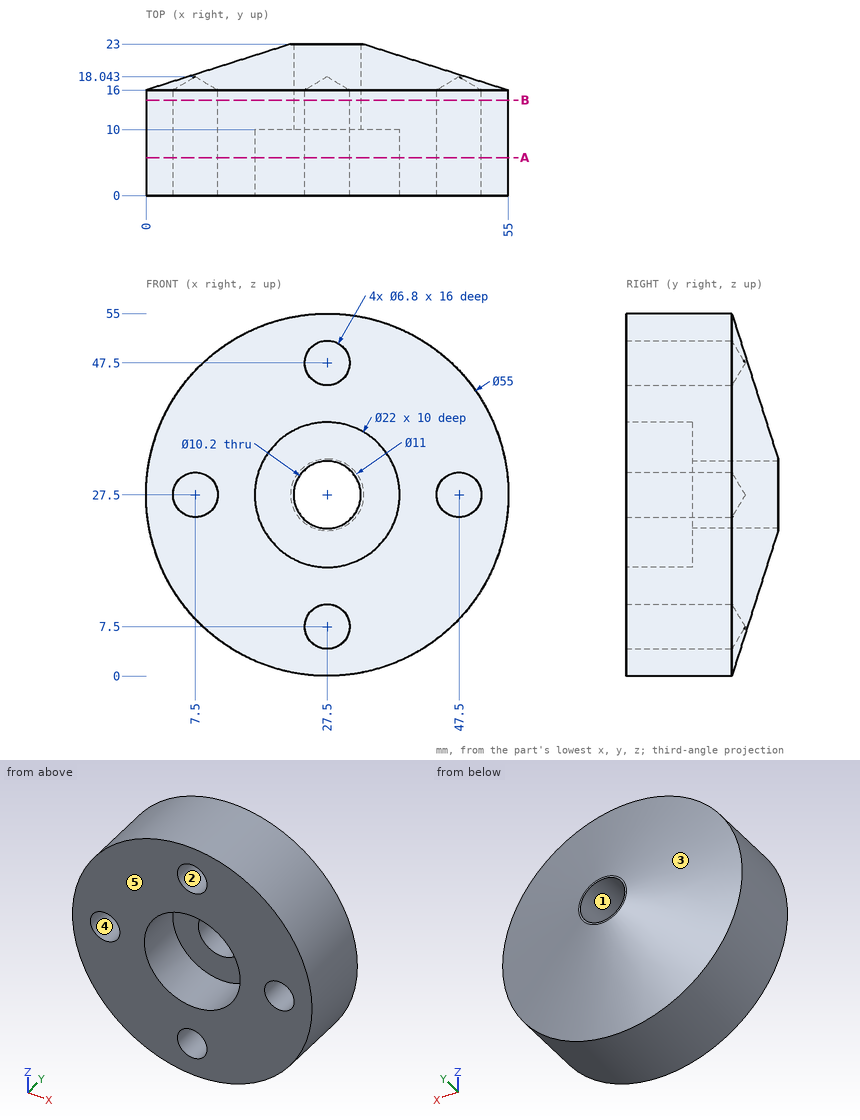
Print and shaded views of the part. All mm, measured from the part's lowest x, y and z. A direction names the side the tool comes from. Give positions to 0.01 mm unless a question says otherwise; leave off trailing zeros. Loops run counter-clockwise (first coordinate to the right, second up) from the corner with the lowest first, then second, coordinate; pieces in that order, holes last. Notation, with made-up numbers: (59, -11.5) - (73, -11.5) arc R19 ccw to (73, 2.5) - close; hole circle Ø8 at (62, -25). An arc over 180 degrees is marked (long way). One line per item, written item: value. Start each with the question number.
1. Pull direction X, two halves, no side cores. Call the marked faces 3, 4 and 5: pulls with the +X half, pulls with the -X half, needs draft (parallel to the pull), parting line crosses it, or undercut.
2. Which spindle directions (+Z, -Z, +X, -X, +Y, -Y) get a long thin tool onto all of the face, cutting with end or side? Do the marked faces 1 and 2. Say none if no direction does.
3. Slice it at A-A (y = 5.75). List the corners of the cut face in (x, z), plus the area to 3 significant figures.
4. Pin check, flat tips, straight feed: pin 1 (1.5 mm diameter, centred on x = 31, z = 39.5, fed in from -Y); pin 2 (9 mm diameter, centred on x = 47.5, z = 27.5, fed in from +Y); pin 3 (3 mm diameter, centred on x = 15.5, y = 12.5, fed in from -Z); pin 4 (6 mm diameter, centred on x = 37, y = 5, fed in from -Z). Stop position of each tip, or through.
5. Probe L1, parallel to Z at x = 27.5, y = 6; L2, parallel to X at y = 11.5, z = 27.5; L3, parallel to X at y = 7.75, z = 5.5. List the from-to ranges inside material, lowest first. Write a range as from..to.
6. Slice it at B-B (y = 14.5). List the corners of the cut face in (x, z).
Solution:
1. face 3: parting line crosses it
1. face 4: undercut
1. face 5: needs draft
2. face 1: +Y, -Y
2. face 2: -Y
3. outline: circle Ø55 at (27.5, 27.5); hole circle Ø6.8 at (7.5, 27.5); hole circle Ø22 at (27.5, 27.5); hole circle Ø6.8 at (27.5, 7.5); hole circle Ø6.8 at (27.5, 47.5); hole circle Ø6.8 at (47.5, 27.5)
3. area: 1,850 mm^2
4. pin 1: stops at y = 0
4. pin 2: stops at y = 19.82
4. pin 3: stops at z = 2.08
4. pin 4: stops at z = 0.78
5. L1: z = 0..4.1, 10.9..16.5, 38.5..44.1, 50.9..55
5. L2: x = 0..4.1, 10.9..22.4, 32.6..44.1, 50.9..55
5. L3: x = 11..24.75, 30.25..44
6. outline: circle Ø55 at (27.5, 27.5); hole circle Ø6.8 at (7.5, 27.5); hole circle Ø10.2 at (27.5, 27.5); hole circle Ø6.8 at (27.5, 7.5); hole circle Ø6.8 at (27.5, 47.5); hole circle Ø6.8 at (47.5, 27.5)
